Model file for the job. Use its own axes, mm. Face numbers are marked on the shaded views. A direction names the side the tool comes from. Coordinates: 2 decimals unless noted, no trailing zeros. Write each loop counter-clockwise with the first axis right and the second up, starting at its lowest first coordinate (ties: lowest second). Pieces come first, ordered by that corner, then holes.
Q1. Band-saw the part on B-B, the plane x = -4.5. Write the cut outline in (y, z), plus the area to 3 significant figures.
Q2. Pull direction Z, two halves, no side cores. Call the marked faces 3, 4 and 5: released by +Z, released by -Z, zero draft, split by the parting line, or undercut.
Q3. Band-saw the part on C-C, the plane y = 2.75. Write the cut outline in (x, z).
Q4. Band-saw the part on D-D, the plane x = 6. Write the cut outline in (y, z).
Q5. Drill centre lines: probe 1 along Z at (x, y) = (0, 2.5); probe 2 along Z at (x, y) = (-3.5, 7.25); probe 3 along X at (y, z) = (9.75, 1.5). Where is each one in solid material? Low to high.
Q6. Which spindle directions (+Z, -Z, +X, -X, +Y, -Y) get a long thin tool onto all of the face, cutting with end or side? Do the marked faces 1 and 2. Say none if no direction does.
Q7. Pin check, flat tips, straight feed: P1, Ø1, axis at x = -4, y = 1.5, coming from the -Z side; P2, Ø6, axis at x = -5, y = 5, coming from the -Z side; P3, Ø3, axis at y = 7, z = 2.5, coming from the +X side. Stop position of each tip, or through.
Q8. Band-saw the part on A-A, the plane z = -2. Write the cut outline in (x, y).
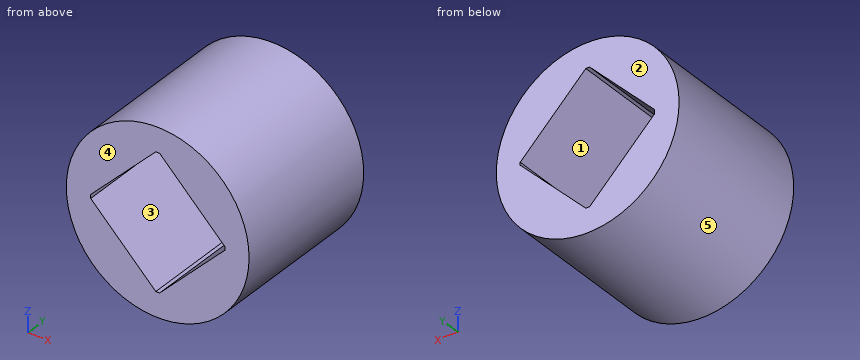
Autodesk Inventor part; units mm, degrees
ref_plane "YZ Plane" through (0, 0, 0) normal (1, 0, 0) x (0, 1, 0)
ref_plane "XZ Plane" through (0, 0, 0) normal (0, 1, 0) x (-1, 0, 0)
ref_plane "XY Plane" through (0, 0, 0) normal (0, 0, 1) x (1, 0, 0)
sketch "Эскиз1" plane through (0, 0, 0) normal (0, 1, 0) x (-1, 0, 0)
  line L0 (-0.1311, -5.5) -> (-5.5, -0.1311)
  line L1 (-5.5, 0.1311) -> (-0.1311, 5.5)
  line L2 (0.1311, 5.5) -> (5.5001, 0.131)
  line L3 (5.5001, -0.131) -> (0.1311, -5.5)
  line L4 (-5.5, 0.131) -> (-5.5, -0.1311)
  line L5 (5.5001, 0.131) -> (5.5001, -0.131)
  line L6 (-0.131, 5.5) -> (0.1311, 5.5)
  line L7 (0.1311, -5.5) -> (-0.1311, -5.5)
  circle A0 centre (0, 0) radius 7.5
extrude "Выдавливание1" add sketch "Эскиз1" along normal blind 13 contours L0 L4 L1 L6 L2 L5 L3 L7 | A0
sketch "Эскиз2" plane through (0, 0, 0) normal (0, -1, 0) x (1, 0, 0)
  circle A0 centre (0, 0) radius 7.5
  line L0 (0.1555, 5.5004) -> (5.5383, 0.1184)
  line L1 (5.5386, -0.1173) -> (0.1571, -5.4996)
  line L2 (-0.156, -5.4999) -> (-5.4995, -0.1573)
  line L3 (-5.4998, 0.1561) -> (-0.0021, 5.6547)
  line L4 (5.5383, 0.1184) -> (5.5386, -0.1173)
  line L5 (-5.4995, -0.1573) -> (-5.4998, 0.1561)
  line L6 (0.1555, 5.5004) -> (-0.1567, 5.5001)
  line L7 (-0.156, -5.4999) -> (0.1571, -5.4996)
  dimension "d4" = 8
  dimension "d5" = 11
extrude "Выдавливание2" cut sketch "Эскиз2" against normal blind 13 contours L0 L4 L1 L7 L2 L5 L3 L6
Answer sheet:
1. outline: (0, -6) - (13, -6) - (13, -1.16) - (0, -1.16) - close; (0, 1.16) - (13, 1.16) - (13, 6) - (0, 6) - close
1. area: 126 mm2
2. face 3: undercut
2. face 4: zero draft
2. face 5: split by the parting line
3. outline: circle Ø15 at (0, 0); hole (-5.5, -0.16) - (-0.16, -5.5) - (0.16, -5.5) - (5.54, -0.12) - (5.54, 0.12) - (0.16, 5.5) - (-0.16, 5.5) - (-5.5, 0.16) - close
4. outline: (0, -4.5) - (13, -4.5) - (13, 4.5) - (0, 4.5) - close
5. probe 1: z = -7.5 to -5.5, 5.5 to 7.5
5. probe 2: z = -6.63 to -2.16, 2.16 to 6.63
5. probe 3: x = -7.35 to -4.16, 4.16 to 7.35
6. face 1: +Y, -Y
6. face 2: +Z, -Z, +X, -X, +Y
7. P1: stops at z = -6.63
7. P2: stops at z = -7.23
7. P3: stops at x = 7.43
8. outline: (-7.23, 0) - (-3.66, 0) - (-3.66, 13) - (-7.23, 13) - close; (3.66, 0) - (7.23, 0) - (7.23, 13) - (3.66, 13) - close
